```python
from build123d import *

# Parameters (mm, degrees)
SKETCH1_W                = 12.7
SKETCH1_H                = 25.4
BOSS_EXTRUDE1_DEPTH      = 3.175
BOSS_EXTRUDE3_DEPTH      = 2.54
BOSS_EXTRUDE3_DEPTH_BACK = 15.24
SKETCH2_R                = 0.635
BOSS_EXTRUDE5_DEPTH      = 2.54
BOSS_EXTRUDE5_DEPTH_BACK = 15.24
SKETCH6_R                = 0.635
SKETCH7_W                = 5.08
SKETCH7_H                = 0.254
CUT_EXTRUDE1_DEPTH       = 30.790908429


with BuildPart() as part:
    # Sketch1 → Boss-Extrude1 (new body)
    with BuildSketch(Plane.XY):
        with Locations((6.35, 12.7)):
            Rectangle(SKETCH1_W, SKETCH1_H)
    extrude(amount=BOSS_EXTRUDE1_DEPTH)

    # Sketch2 → Boss-Extrude3 (add, two sides: drawn at the far end of the back side and taken through both)
    with BuildSketch(Plane(origin=(12.7, 0, 0), x_dir=(0, 0, -1), z_dir=(1, 0, 0)).offset(-BOSS_EXTRUDE3_DEPTH_BACK)):
        with Locations((-1.5875, 22.225)):
            Circle(SKETCH2_R)
    extrude(amount=BOSS_EXTRUDE3_DEPTH + BOSS_EXTRUDE3_DEPTH_BACK)

    # Sketch6 → Boss-Extrude5 (add, two sides: drawn at the far end of the back side and taken through both)
    with BuildSketch(Plane(origin=(12.7, 0, 0), x_dir=(0, 0, -1), z_dir=(1, 0, 0)).offset(-BOSS_EXTRUDE5_DEPTH_BACK)):
        with Locations((-1.5875, 3.175)):
            Circle(SKETCH6_R)
    extrude(amount=BOSS_EXTRUDE5_DEPTH + BOSS_EXTRUDE5_DEPTH_BACK)

    # Sketch7 → Cut-Extrude1 (cut, through all)
    with BuildSketch(Plane(origin=(0, 25.4, 0), x_dir=(1, 0, 0), z_dir=(0, 1, 0))):
        with Locations((6.35, -2.403553661)):
            Rectangle(SKETCH7_W, SKETCH7_H)
    extrude(amount=-CUT_EXTRUDE1_DEPTH, mode=Mode.SUBTRACT)


solid = part.part
```
Check sheet for the modelled part. Datum: model origin and axes. Units: mm. A direction names the side the tool comes from. Coordinates: 2 decimals unless noted, no trailing zeros. Order: outer loops, then holes, each group sorted by start corner. A loop starts at its lowest first (then second) coordinate and runs counter-clockwise, first axis right, second up. Notation, with made-up numbers: (17.25, 32) -> (71.25, 32) arc R13 ccw to (71.25, 57) -> close; hole circle Ø5 at (56.5, 31). An arc over 180 degrees is marked (long way). Write each question's results on one line, items separated by ' | '. Start each with the question number.
1) Depth check by flat-ended pin: pin 1 (1.6 mm diameter, centred on y = 11, z = 1.5, fed in from -X); pin 2 (8 mm diameter, centred on x = 4.5, y = 20.5, fed in from -Z). Enter the tip coordinate at first touch or a pass-through.
2) Section check B-B (y = 8.5). Enter the section's corners in (x, z) (3 decimals), and give its area (3 significant figures).
3) Section check A-A (x = 7). Enter the section's corners in (y, z) (3 decimals).
4) Section check D-D (y = 22.5). Enter the section's corners in (x, z) (3 decimals).
5) Material ranges on line 1 along X through (y, z) = (13.5, 2.5); line 2 along Z through (x, y) = (5.75, 17.5) (3 decimals); line 3 along X through (y, z) = (23.75, 0.8), recorded low to high.
6) Draft check along Z on faces 4 (the face through (6, 13, 2.277)), 5 (the face through (-1.288, 22.855, 1.67)), 6 (the face through (6, 0, 2)), 7 (the face through (6, 13, 2.531)). Enter one of: pulls with the +Z half, pulls with the -Z half, needs draft (parallel to the pull), parting line crosses it, or undercut.
7) Set-up check for faces 1 (the face through (-1.3, 3.8, 1.7)), 2 (the face through (-2.54, 22, 2)), 3 (the face through (14, 3.8, 1.7)): record each of +Z, -Z, +X, -X, +Y, -Y from which the full face is reachable in a straight line by a thin tool's end or side.
8) Section check C-C (z = 1.55). Enter the section's corners in (x, y).
Checked values:
1) pin 1: x = 0 | pin 2: z = 0
2) outline: (0, 0) -> (12.7, 0) -> (12.7, 3.175) -> (0, 3.175) -> close; hole (3.81, 2.277) -> (8.89, 2.277) -> (8.89, 2.531) -> (3.81, 2.531) -> close | area: 39.0 mm²
3) outline: (0, 0) -> (25.4, 0) -> (25.4, 2.277) -> (0, 2.277) -> close; (0, 2.531) -> (25.4, 2.531) -> (25.4, 3.175) -> (0, 3.175) -> close
4) outline: (-2.54, 1.015) -> (0, 1.015) -> (0, 0) -> (12.7, 0) -> (12.7, 1.015) -> (15.24, 1.015) -> (15.24, 2.16) -> (12.7, 2.16) -> (12.7, 3.175) -> (0, 3.175) -> (0, 2.16) -> (-2.54, 2.16) -> close; hole (3.81, 2.277) -> (8.89, 2.277) -> (8.89, 2.531) -> (3.81, 2.531) -> close
5) line 1: 0 to 3.81, 8.89 to 12.7 | line 2: 0 to 2.277, 2.531 to 3.175 | line 3: 0 to 12.7
6) face 4: undercut | face 5: parting line crosses it | face 6: needs draft | face 7: undercut
7) face 1: -X | face 2: +Z, -Z, -X, +Y, -Y | face 3: +X
8) outline: (-2.54, 2.54) -> (0, 2.54) -> (0, 0) -> (12.7, 0) -> (12.7, 2.54) -> (15.24, 2.54) -> (15.24, 3.81) -> (12.7, 3.81) -> (12.7, 21.59) -> (15.24, 21.59) -> (15.24, 22.86) -> (12.7, 22.86) -> (12.7, 25.4) -> (0, 25.4) -> (0, 22.86) -> (-2.54, 22.86) -> (-2.54, 21.59) -> (0, 21.59) -> (0, 3.81) -> (-2.54, 3.81) -> close
